Verification items for the finished model (mm, model axes). A direction names the side the tool comes from. Give positions to 0.01 mm unless a question says otherwise; leave off trailing zeros. Order: outer loops, then holes, each group sorted by start corner. A loop starts at its lowest first (then second) coordinate and runs counter-clockwise, first axis right, second up. Notation, with made-up numbers: (-19, 50) -> (3, 50) arc R25 cw to (3, 82) -> close; hole circle Ø11 at (27.25, 50). An arc over 180 degrees is marked (long way). Return JSON: item names as keys, results as strings. Group by question number.
(1) Cross-section at B-B on z = -5.15. Enter the section's corners in (x, y).
(2) Tool access check on faces 1 (the face through (0.85, 0.99, -5.18)), 2 (the face through (0, 3, -8)), 3 (the face through (-11.3, 0.7, 8.4)), 4 (the face through (-10.75, 0.93, 7.09)), 5 (the face through (3, 2, 0)). Record the directions out of +Z, -Z, +X, -X, +Y, -Y that give a thin tool (end or side, any length) a straight path to the whole face; none if there is none.
(3) Cross-section at D-D on y = 3.8. Enter the section's corners in (x, z).
(4) Depth check by flat-ended pin: pin 1 Ø1.5 at (x, y) = (-6.5, 2) entering from +Z; pin 2 Ø6.5 at (x, z) = (-2, -2) entering from +Y; pin 3 Ø6 at (x, z) = (-1, -3.5) entering from +Y. Enter the tip coordinate at first touch or a pass-through.
(5) Cross-section at C-C on x = 2. Enter the section's corners in (y, z), then the cut area to 3 significant figures.
(6) Cross-section at A-A on x = -6. Enter the section's corners in (y, z).
(7) Thickness scan on line 1 along Z through (x, y) = (-6, 1.5); line 2 along Z through (x, y) = (-3.5, 2.45); line 3 along Y through (x, z) = (-3.75, -0.5). Record the ranges inside material, lowest first.
Autodesk Inventor part; units mm, degrees
ref_plane "YZ Plane" through (0, 0, 0) normal (1, 0, 0) x (0, 1, 0)
ref_plane "XZ Plane" through (0, 0, 0) normal (0, 1, 0) x (-1, 0, 0)
ref_plane "XY Plane" through (0, 0, 0) normal (0, 0, 1) x (1, 0, 0)
sketch "Sketch3" plane through (0, 0, 0) normal (0, 1, 0) x (-1, 0, 0)
  line L0 (11.3, 9) -> (-11.3, 9)
  line L1 (-11.3, 9) -> (-11.3, -9)
  line L2 (-11.3, -9) -> (11.3, -9)
  line L3 (11.3, -9) -> (11.3, 9)
  line L4 (11.3, 9) -> (-11.3, -9) construction
  line L5 (-11.3, 9) -> (11.3, -9) construction
  line L6 (11.3, 5.15) -> (0.3, 5.15) construction
  line L7 (11.3, 6.3) -> (0.3, 6.3)
  line L8 (0.3, 4) -> (11.3, 4)
  arc A0 (11.3, 4) -> (11.3, 6.3) centre (11.3, 5.15) ccw
  arc A1 (0.3, 6.3) -> (0.3, 4) centre (0.3, 5.15) ccw
  line L9 (11.3, -5.15) -> (0.3, -5.15) construction
  line L10 (11.3, -4) -> (0.3, -4)
  line L11 (0.3, -6.3) -> (11.3, -6.3)
  arc A2 (11.3, -6.3) -> (11.3, -4) centre (11.3, -5.15) ccw
  arc A3 (0.3, -4) -> (0.3, -6.3) centre (0.3, -5.15) ccw
  point P0 (0, 0)
  point P1 (5.8, 5.15)
  point P2 (5.8, -5.15)
  dimension "d4" = 18
  dimension "d5" = 22.6
  dimension "d6" = 11
  dimension "d7" = 11
  dimension "d8" = 2.3
  dimension "d9" = 2.3
  dimension "d10" = 12.6
  dimension "d11" = 6.3
extrude "Extrusion3" add sketch "Sketch3" along normal blind 3 contours L3 L7 A1 L8 L10 A3 L11 L2 L1 L0
sketch "Sketch4" plane through (-11.3, 0, -4) normal (-1, 0, 0) x (0, 0, 1)
  line L0 (-2.3, 3) -> (0, 3)
  line L1 (10.3, 0) -> (10.3, 3)
  line L2 (-2.3, 3) -> (10.3, 3)
  line L3 (10.3, 3) -> (10.3, 2)
  line L4 (10.3, 2) -> (-2.3, 2)
  line L5 (-2.3, 2) -> (-2.3, 3)
  point P0 (4, 0)
  dimension "d14" = 1
extrude "Extrusion4" cut sketch "Sketch4" against normal blind 30
chamfer "Chamfer1" distance 2.5 angle 45 1 edges at (11.3, 3, -7.65)
sketch "Sketch5" plane through (0, 0, 0) normal (0, 0, 1) x (1, 0, 0)
  circle A0 centre (-10.7, 3) radius 1.5
  line L0 (11.3, 0) -> (11.3, 0.5)
  line L1 (-11.7607, 1.9393) -> (-9.8213, 0)
  line L2 (-11.3, 0) -> (11.3, 0)
  line L3 (-9.6393, 4.0607) -> (-7.5787, 2)
  line L4 (-0.3, 2) -> (-11.3, 2)
  line L5 (-7.5787, 2) -> (-9.8213, 0)
  point P0 (0, 0)
  point P1 (-9.582, 2)
  dimension "d20" = 3
  dimension "d21" = 3
  dimension "d22" = 22
  dimension "d23" = 135
  dimension "d24" = 135
extrude "Extrusion5" add sketch "Sketch5" along normal mid plane 18
sketch "Sketch6" plane through (-11.7607, 1.9393, 9) normal (-0.7071, -0.7071, 0) x (-0.7071, 0.7071, 0)
  line L0 (6.2129, 16.9) -> (-25.5876, 16.9)
  line L1 (-25.5876, 16.9) -> (-25.5876, 1.1)
  line L2 (-25.5876, 1.1) -> (6.2129, 1.1)
  line L3 (6.2129, 1.1) -> (6.2129, 16.9)
  line L4 (6.2129, 16.9) -> (-25.5876, 1.1) construction
  line L5 (-25.5876, 16.9) -> (6.2129, 1.1) construction
  point P0 (-9.6874, 9)
  dimension "d27" = 15.8
extrude "Extrusion6" cut sketch "Sketch6" along normal blind 10
extrude "Extrusion7" add sketch "Sketch5" along normal mid plane 21.2 contours A0
sketch "Sketch7" plane through (0, 0, 0) normal (0, -1, 0) x (1, 0, 0)
  line L0 (-11.3, -9) -> (-11.7607, -9)
  line L1 (-11.3, -9) -> (-10.9536, -9.6)
  line L2 (-10.9536, -9.6) -> (-10.6536, -9.6)
  line L3 (-10.6536, -9.6) -> (-10.3072, -9)
  line L4 (-9.2, -9) -> (-11.7607, -9)
  point P0 (0, 0)
  point P1 (-9.6393, -9)
  dimension "d32" = 9.6
  dimension "d33" = 60
  dimension "d34" = 60
  dimension "d35" = 0.3
extrude "Extrusion8" add sketch "Sketch7" against normal up to next
mirror "Mirror1" about plane through (0, 0, 0) normal (0, 0, 1) of "Extrusion8"
sketch "Sketch8" plane through (0, 0, 0) normal (0, -1, 0) x (1, 0, 0)
  line L0 (-9.8213, -6.3) -> (-0.3, -6.3)
  line L1 (-0.3, -6.3) -> (-24.4848, -6.3)
  line L2 (-24.4848, -6.3) -> (-24.4848, -4)
  line L3 (-24.4848, -4) -> (-0.3, -4)
  line L4 (-0.3, -4) -> (-0.3, -6.3)
  line L5 (-0.3, 4) -> (-7.5787, 4)
  line L6 (-0.3, 4) -> (-23.0411, 4)
  line L7 (-23.0411, 4) -> (-23.0411, 6.3)
  line L8 (-23.0411, 6.3) -> (-0.3, 6.3)
  line L9 (-0.3, 6.3) -> (-0.3, 4)
  line L10 (-0.3, -4) -> (-9.8213, -4)
  line L11 (-0.3, 6.3) -> (-9.8213, 6.3)
  point P0 (0, 0)
extrude "Extrusion9" cut sketch "Sketch8" against normal blind 10
equation "\"d7\" = d6"
equation "\"d9\" = d8"
Verdict:
{
 "1": {"outline": "(0.85, 0) -> (11.3, 0) -> (11.3, 0.5) -> (9.8, 2) -> (0.85, 2) -> close"},
 "2": {"face 1": "-X, +Y, -Y", "face 2": "+Z, -Z, +X, +Y", "face 3": "+Z, -Z, -X, -Y", "face 4": "-X, -Y", "face 5": "+X, +Y"},
 "3": {"outline": "(-11.97, -10.6) -> (-9.43, -10.6) -> (-9.43, -9) -> (-9.38, -9) -> (-9.38, -6.3) -> (-11.97, -6.3) -> close; (-11.97, -4) -> (-9.38, -4) -> (-9.38, 4) -> (-11.97, 4) -> close; (-11.97, 6.3) -> (-9.38, 6.3) -> (-9.38, 9) -> (-9.43, 9) -> (-9.43, 10.6) -> (-11.97, 10.6) -> close"},
 "4": {"pin 1": "z = 9", "pin 2": "y = 2", "pin 3": "y = 3"},
 "5": {"outline": "(0, -9) -> (3, -9) -> (3, -6.3) -> (2, -6.3) -> (2, 6.3) -> (3, 6.3) -> (3, 9) -> (0, 9) -> close", "area": "41.4 mm²"},
 "6": {"outline": "(0, -9) -> (3, -9) -> (3, -6.3) -> (0, -6.3) -> close; (0, -4) -> (2, -4) -> (2, 4) -> (0, 4) -> close; (0, 6.3) -> (3, 6.3) -> (3, 9) -> (0, 9) -> close"},
 "7": {"line 1": "-9 to -6.3, -4 to 4, 6.3 to 9", "line 2": "-9 to -6.3, 6.3 to 9", "line 3": "0 to 2"}
}
